Autodesk Inventor part; units mm, degrees
ref_plane "YZ Plane" through (0, 0, 0) normal (1, 0, 0) x (0, 1, 0)
ref_plane "XZ Plane" through (0, 0, 0) normal (0, 1, 0) x (-1, 0, 0)
ref_plane "XY Plane" through (0, 0, 0) normal (0, 0, 1) x (1, 0, 0)
sketch "Sketch1" plane through (0, 0, 0) normal (1, 0, 0) x (0, 1, 0)
  line L0 (0, 0) -> (0, -266.7) construction
  line L1 (0, 0) -> (15.875, 0) construction
  line L2 (0, 0) -> (-15.875, 0) construction
  line L3 (0, -266.7) -> (15.875, -266.7) construction
  line L4 (0, -266.7) -> (15.875, -266.7) construction
  line L5 (0, -266.7) -> (-15.875, -266.7) construction
  line L6 (0, -266.7) -> (15.875, -266.7) construction
  arc A0 (15.875, 0) -> (-15.875, 0) centre (0, 0) ccw
  line L7 (15.875, 0) -> (15.875, -266.7)
  line L8 (-15.875, 0) -> (-15.875, -266.7)
  arc A1 (-15.875, -266.7) -> (15.875, -266.7) centre (0, -266.7) ccw
  line L9 (22.225, -266.7) -> (22.225, 0)
  arc A2 (22.225, 0) -> (-22.225, 0) centre (0, 0) ccw
  line L10 (-22.225, 0) -> (-22.225, -266.7)
  arc A3 (-22.225, -266.7) -> (22.225, -266.7) centre (0, -266.7) ccw
  dimension "d0" = 266.7
  dimension "d3" = 15.875
  dimension "d4" = 15.875
  dimension "d5" = 15.875
  dimension "d6" = 0
  dimension "d7" = 15.875
  dimension "d8" = 180
  dimension "d9" = 15.875
  dimension "d10" = 15.875
  dimension "d11" = 6.35
extrude "Extrusion1" add sketch "Sketch1" along normal blind 6.35
properties part number "chain"
Geometry check sheet. Reference: the model listing, model coordinates, mm. A direction names the side the tool comes from. Round coordinates to 2 decimals unless told otherwise and drop trailing zeros. Loops run counter-clockwise (first coordinate to the right, second up) from the corner with the lowest first, then second, coordinate; pieces in that order, holes last. Notation, with made-up numbers: (13, 12.25) -> (22, 12.25) arc R33 cw to (22, 42.25) -> close; hole circle Ø9 at (50, 71.5). An arc over 180 degrees is marked (long way). Use a Markdown table: item, result.
(1) Set-up check for faces 1 (the cylindrical face through (3.13, 0.49, -288.92)), 2 (the flat face through (3, 15.875, -131)): record each of +Z, -Z, +X, -X, +Y, -Y from which the full face is reachable in a straight line by a thin tool's end or side.
Calculated:
| item | result |
|---|---|
| face 1 | -Z, +X, -X |
| face 2 | +X, -X |
(2) Scan lines: probe 1 along Y at (x, z) = (3.25, -179) (3 decimals); probe 2 along Z at (x, y) = (4.5, 0) (3 decimals); probe 3 along Z at (x, y) = (1, 14.5). Record each from-to range of solid material in increasing order.
Calculated:
| item | result |
|---|---|
| probe 1 | -22.225 to -15.875, 15.875 to 22.225 |
| probe 2 | -288.925 to -282.575, 15.875 to 22.225 |
| probe 3 | -283.54 to -273.16, 6.46 to 16.84 |
(3) Go/stop test with flat-tipped pins: P1, Ø2, axis at x = 2.5, y = 2, coming from the -Z side; P2, Ø1.5, axis at x = 3.5, y = 4.5, coming from the +Z side; P3, Ø3, axis at x = 3.5, y = 7, coming from the +Z side. Record where each tip stops, or that it passes through.
Calculated:
| item | result |
|---|---|
| P1 | z = -288.9 |
| P2 | z = 21.91 |
| P3 | z = 21.53 |
(4) Mould release check, pull along X, two halves, no side actions. Record for faces 3 (the flat face through (6.35, -17, -133)), 4 (the flat face through (0, -17, -133)), 5 (the cylindrical face through (3.13, 0.35, -282.57)): released by +X, released by -X, zero draft, split by the parting line, or undercut.
Calculated:
| item | result |
|---|---|
| face 3 | released by +X |
| face 4 | released by -X |
| face 5 | zero draft |
(5) Sectioned sample at B-B (z = -31). Enter the section's corners in (x, y) (3 decimals), then the cut area to 3 significant figures.
Calculated:
| item | result |
|---|---|
| outline | (0, -22.225) -> (6.35, -22.225) -> (6.35, -15.875) -> (0, -15.875) -> close; (0, 15.875) -> (6.35, 15.875) -> (6.35, 22.225) -> (0, 22.225) -> close |
| area | 80.6 mm² |
(6) Sectioned sample at C-C (x = 3.5). Enter the section's corners in (y, z) (3 decimals).
Calculated:
| item | result |
|---|---|
| outline | (-22.225, -266.7) arc R22.225 ccw to (22.225, -266.7) -> (22.225, 0) arc R22.225 ccw to (-22.225, 0) -> close; hole (-15.875, -266.7) arc R15.875 ccw to (15.875, -266.7) -> (15.875, 0) arc R15.875 ccw to (-15.875, 0) -> close |
(7) Sectioned sample at A-A (y = 0). Enter the section's corners in (x, z) (3 decimals), then the cut area to 3 significant figures.
Calculated:
| item | result |
|---|---|
| outline | (0, -288.925) -> (6.35, -288.925) -> (6.35, -282.575) -> (0, -282.575) -> close; (0, 15.875) -> (6.35, 15.875) -> (6.35, 22.225) -> (0, 22.225) -> close |
| area | 80.6 mm² |
